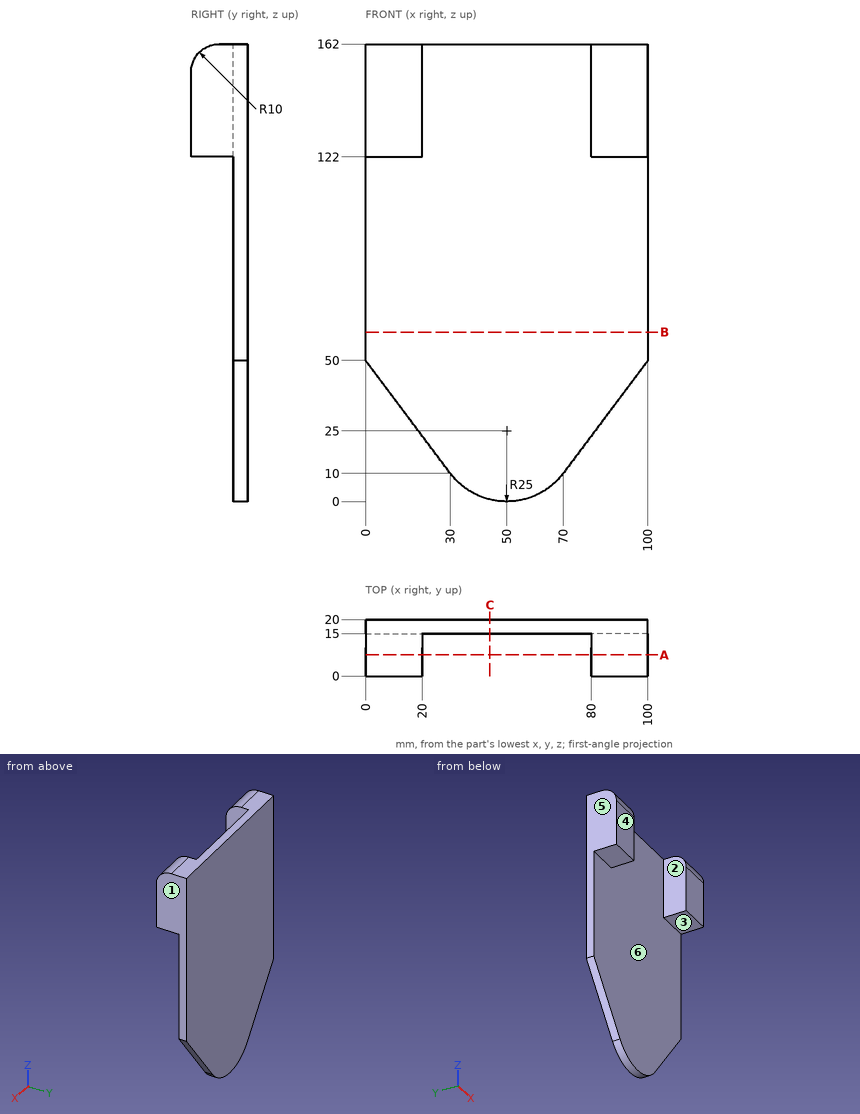
Design review of the part shown in the three views and the two pictorial views. Dimensions are in mm from the part's minimum x, y and z. A direction names the side the tool comes from. Round coordinates to 2 decimals unless told otherwise and drop trailing zeros. Write each loop counter-clockwise with the first axis right and the second up, starting at its lowest first coordinate (ties: lowest second). Pieces come first, ordered by that corner, then holes.
Item 1: Consider section B-B on z = 60. Give the boundary of the cut face in (x, y).
Item 2: Consider section A-A on y = 7.5. Give the boundary of the cut face in (x, z).
Item 3: Wall thickness on L1, parallel to Y at x = 90, z = 119; L2, parallel to X at y = 14.5, z = 155.5; L3, parallel to Z at x = 7.5, y = 13.5: over which ranges is each line inside the solid? List them lowest first.
Item 4: For pin 1 Ø7.5 at (x, y) = (89.5, 5) entering from -Z; pin 2 Ø6 at (x, y) = (74.5, 3) entering from +Z; pin 3 Ø12 at (y, z) = (11, 140) entering from -X; pin 4 Ø12 at (y, z) = (14.5, 20) entering from +X, all flat-tipped, find the tip position at first contact; note any pin that passes through.
Item 5: For the marked faces 1, 2 and 3, list the 3-axis set-ups (+Z, -Z, +X, -X, +Y, -Y) from which the entire face can be reached by the end or side of a thin tool; tool diameter is ignored.
Item 6: Consider section C-C on x = 44. Give the boundary of the cut face in (y, z), and give its area (3 significant figures).
Item 7: Draft analysis for pull direction X (two halves, no side actions). For the marked faces 4, 5 and 6, state which applies: released by +X, released by -X, zero draft, split by the parting line, or undercut.
Check values:
1. outline: (0, 15) - (100, 15) - (100, 20) - (0, 20) - close
2. outline: (0, 122) - (20, 122) - (20, 161.68) - (0, 161.68) - close; (80, 122) - (100, 122) - (100, 161.68) - (80, 161.68) - close
3. L1: y = 15 to 20
3. L2: x = 0 to 20, 80 to 100
3. L3: z = 122 to 162
4. pin 1: stops at z = 122
4. pin 2: passes through
4. pin 3: stops at x = 0
4. pin 4: stops at x = 81.98
5. face 1: +Z, -Z, +X, +Y, -Y
5. face 2: +Z, -Z, -Y
5. face 3: -Z, +X, -X, -Y
6. outline: (15, 0.73) - (20, 0.73) - (20, 162) - (15, 162) - close
6. area: 806 mm2
7. face 4: zero draft
7. face 5: released by -X
7. face 6: undercut
